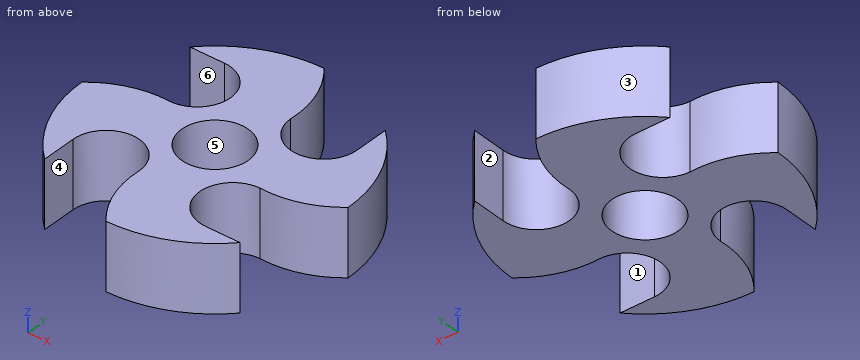
Autodesk Inventor part; units mm, degrees
ref_plane "YZ Plane" through (0, 0, 0) normal (1, 0, 0) x (0, 1, 0)
ref_plane "XZ Plane" through (0, 0, 0) normal (0, 1, 0) x (-1, 0, 0)
ref_plane "XY Plane" through (0, 0, 0) normal (0, 0, 1) x (1, 0, 0)
sketch "Sketch1" plane through (0, 0, 0) normal (0, 0, 1) x (1, 0, 0)
  circle A0 centre (0, 0) radius 12.7
  dimension "d0" = 25.4
extrude "Extrusion1" add sketch "Sketch1" along normal blind 6.35
sketch "Sketch2" plane through (0, 0, 6.35) normal (0, 0, 1) x (1, 0, 0)
  circle A0 centre (0, 0) radius 12.7
  arc A1 (-6.4006, 2.2157) -> (-6.1091, 8.5523) centre (-6.1091, 5.3773) ccw
  line L0 (-6.1091, 8.5523) -> (-9.3887, 8.5523)
  arc A2 (-6.1091, 2.2023) -> (-12.7, 0) centre (-6.6809, -7.0502) ccw
  dimension "d3" = 6.35
extrude "Extrusion2" cut sketch "Sketch2" against normal blind 50.8 contours L0 A1 A2 A0 picked at (-7.9, 5.5911)
pattern_circular "Circular Pattern1" count 4 over 360 about axis through (0, 0, -10) along (0, 0, 1) of "Extrusion2"
sketch "Sketch3" plane through (0, 0, 6.35) normal (0, 0, 1) x (1, 0, 0)
  arc A0 (12.7, 0) -> (8.5523, 9.3887) centre (0, 0) ccw
  circle A1 centre (0, 0) radius 3.175
  dimension "d9" = 6.35
extrude "Extrusion3" cut sketch "Sketch3" against normal blind 50.8
properties part number "ratchet"
For this review, take the finished solid that the model builds, in its own axes (mm). Face numbers are marked on the shaded views. A direction names the side the tool comes from. Give positions to 0.01 mm unless a question says otherwise; leave off trailing zeros. Write each loop counter-clockwise with the first axis right and the second up, starting at its lowest first coordinate (ties: lowest second). Pieces come first, ordered by that corner, then holes. Notation, with made-up numbers: M 2,81 L 22,81 A21 ccw 22,93 Z; hole C -13,10.25 d2. An arc over 180 degrees is marked long. Answer as a JSON object with one key per item and string values. Group by question number.
Item 1: Consider section C-C on z = 5. Write out the cut boundary in (x, y) (3 decimals).
Item 2: For pin 1 Ø1.5 at (y, z) = (-10, 4) entering from -X; pin 2 Ø1 at (x, z) = (-7.5, 4) entering from -Y; pin 3 Ø1.6 at (y, z) = (-7, 2) entering from +X; pin 4 Ø5 at (x, y) = (0, 0) entering from +Z, all flat-tipped, find the tip position at first contact; note any pin that passes through.
Item 3: Consider section B-B on x = -1.5. Write out the cut boundary in (y, z).
Item 4: Tool access review of the marked faces 4, 5 and 6: name each direction out of +Z, -Z, +X, -X, +Y, -Y from which nothing blocks a thin tool from reaching the whole face with its end or side.
Item 5: Consider section D-D on y = -9.75. Write out the cut boundary in (x, z).
Item 6: Consider section A-A on y = 5.75. Write out the cut boundary in (x, z), plus the area to 3 significant figures.
Item 7: For probe 1 along Y at (x, z) = (-4.5, 3); probe 2 along Y at (x, z) = (3.75, 5); probe 3 along X at (y, z) = (6.5, 4.75), list the stretches that pass through material, from the lowest coordinate up. Write a range as [from, to].
Item 8: Draft analysis for pull direction Y (two halves, no side actions). For the marked faces 1, 2 and 3, state which applies: +Y half, -Y half, draft (parallel to the pull), parting line (faces both ways), or undercut.
Check result:
{
 "1": {"outline": "M -12.7,0 A12.7 ccw -8.552,-9.389 L -8.552,-6.109 A3.175 cw -2.202,-6.109 A9.27 ccw 0,-12.7 A12.7 ccw 9.389,-8.552 L 6.109,-8.552 A3.175 cw 6.109,-2.202 A9.27 ccw 12.7,0 A12.7 ccw 8.552,9.389 L 8.552,6.109 A3.175 cw 2.202,6.109 A9.27 ccw 0,12.7 A12.7 ccw -9.389,8.552 L -6.109,8.552 A3.175 cw -6.109,2.202 A9.27 ccw Z; hole C 0,0 d6.35"},
 "2": {"pin 1": "stops at x = -8.7", "pin 2": "stops at y = -4.32", "pin 3": "stops at x = 4.06", "pin 4": "passes through"},
 "3": {"outline": "M -10.26,0 L -2.8,0 L -2.8,6.35 L -10.26,6.35 Z; M 2.8,0 L 12.61,0 L 12.61,6.35 L 2.8,6.35 Z"},
 "4": {"face 4": "+Z, -Z, -Y", "face 5": "+Z, -Z", "face 6": "+Z, -Z, -X"},
 "5": {"outline": "M -1.7,0 L 8.14,0 L 8.14,6.35 L -1.7,6.35 Z"},
 "6": {"outline": "M -2.96,0 L 2.22,0 L 2.22,6.35 L -2.96,6.35 Z; M 8.53,0 L 11.32,0 L 11.32,6.35 L 8.53,6.35 Z", "area": "50.6 mm^2"},
 "7": {"probe 1": "y = [-3.06, 2.64], [8.11, 11.88]", "probe 2": "y = [-12.13, -7.5], [-3.25, 3.38]", "probe 3": "x = [-3.14, 2.22], [8.55, 10.91]"},
 "8": {"face 1": "undercut", "face 2": "draft", "face 3": "+Y half"}
}
